```python
from build123d import *

# Parameters (mm, degrees)
BOSS_EXTRUDE1_DEPTH = 5
CUT_EXTRUDE1_DEPTH  = 5


with BuildPart() as part:
    # Sketch2 → Boss-Extrude1 (new body)
    with BuildSketch(Plane.XY):
        with BuildLine():
            Line((-227.482425682, -83.89157587), (-200.672425682, -83.89157587))
            Line((-200.672425682, -83.89157587), (-200.672425682, -68.99157587))
            Line((-200.672425682, -68.99157587), (-176.574253233, -68.99157587))
            ThreePointArc((-176.574253233, -68.99157587), (-129.684755475, -47.286361961), (-115.892707438, 2.50842413))
            Line((-115.892707438, 2.50842413), (-180.821327591, 2.50842413))
            Line((-180.821327591, 2.50842413), (-227.482425682, -45.84868874))
            Line((-227.482425682, -45.84868874), (-227.482425682, -83.89157587))
        make_face()
    extrude(amount=BOSS_EXTRUDE1_DEPTH)

    # Sketch4 → Cut-Extrude1 (cut)
    with BuildSketch(Plane.XY.offset(5)):
        Polygon((-212.822425682, -83.89157587), (-208.922425682, -83.89157587), (-208.922425682, -81.89157587), (-207.472425682, -81.89157587), (-207.472425682, -78.89157587), (-208.922425682, -78.89157587), (-208.922425682, -70.89157587), (-212.822425682, -70.89157587), (-212.822425682, -78.89157587), (-214.272425682, -78.89157587), (-214.272425682, -81.89157587), (-212.822425682, -81.89157587), align=None)
        Polygon((-222.822425682, -83.89157587), (-218.922425682, -83.89157587), (-218.922425682, -81.89157587), (-217.472425682, -81.89157587), (-217.472425682, -78.89157587), (-218.922425682, -78.89157587), (-218.922425682, -70.89157587), (-222.822425682, -70.89157587), (-222.822425682, -78.89157587), (-224.272425682, -78.89157587), (-224.272425682, -81.89157587), (-222.822425682, -81.89157587), align=None)
    extrude(amount=-CUT_EXTRUDE1_DEPTH, mode=Mode.SUBTRACT)


solid = part.part
```
Could you check a few things on this model? Use its own coordinates, in mm. A direction names the side the tool comes from. Round coordinates to 2 decimals unless told otherwise and drop trailing zeros. Write each loop counter-clockwise with the first axis right and the second up, starting at its lowest first coordinate (ties: lowest second). Pieces come first, ordered by that corner, then holes. Notation, with made-up numbers: M 89.25,10.25 L 118.25,10.25 A8 cw 118.25,23.25 Z; hole C -7.75,-28.5 d11. An arc over 180 degrees is marked long. Write each question's results on one line, items separated by ' | '. Start each with the question number.
1. I'm going to push flat-ended pins straight in: pin 1 Ø1.2 at (x, z) = (-208.5, 2) entering from +Y; pin 2 Ø1 at (y, z) = (-83, 3) entering from +X; pin 3 Ø1.5 at (y, z) = (-62.5, 4) entering from +X. Where does each tip first touch, or does it pass through?
2. Thinking about a two-plate mould opening in X: for faces 5 (the face through (-212.822, -75, 3)), 6 (the face through (-130.17, -47.85, 2.46)), 7 (the face through (-205, -83.892, 2)), which applies, +X half, -X half, draft (parallel to the pull), parting line (faces both ways), or undercut?
3. Imagine slicing it at D-D on y = -15. List the corners of the cut face in (x, z) for me.
4. I need wall thicknesses on L1, parallel to X at y = -73, z = 3.45; L2, parallel to X at y = -69.5, z = 4.6; L3, parallel to Y at x = -217, z = 2.6. Which ranges of each line are inside material? Lowest first, please. Write a range as from..to.
5. On a 3-axis mill with a long thin cutter (end or side, diameter ignored), from which of +Z, -Z, +X, -X, +Y, -Y can I reach the whole of each face in a straight line? I mean faces 1 (the face through (-214.272, -80, 3)), 2 (the face through (-200.672, -77, 2)), 3 (the face through (-221, -70.892, 3)), 4 (the face through (-148, 2.508, 2)). Say none if no direction works.
6. Imagine slicing it at C-C on x = -158. List the corners of the cut face in (y, z) for me, and give its area (3 significant figures).
7. Imagine slicing it at A-A on y = -74. List the corners of the cut face in (x, z) for me.
Result sheet:
1) pin 1: stops at y = -25.55 | pin 2: stops at x = -200.67 | pin 3: stops at x = -147.62
2) face 5: undercut | face 6: +X half | face 7: draft
3) outline: M -197.72,0 L -115.53,0 L -115.53,5 L -197.72,5 Z
4) L1: x = -227.48..-222.82, -218.92..-212.82, -208.92..-200.67 | L2: x = -227.48..-200.67 | L3: y = -83.89..-34.99
5) face 1: +Z, -Z | face 2: +Z, -Z, +X, -Y | face 3: +Z, -Z, -Y | face 4: +Z, -Z, +X, -X, +Y
6) outline: M -66.12,0 L 2.51,0 L 2.51,5 L -66.12,5 Z | area: 343 mm^2
7) outline: M -227.48,0 L -222.82,0 L -222.82,5 L -227.48,5 Z; M -218.92,0 L -212.82,0 L -212.82,5 L -218.92,5 Z; M -208.92,0 L -200.67,0 L -200.67,5 L -208.92,5 Z
